For this review, take the finished solid that the model builds, in its own axes (mm). Give positions to 0.01 mm unless a question says otherwise; leave off trailing zeros. Order: outer loops, then holes, each group sorted by start corner. A loop starts at its lowest first (then second) coordinate and runs counter-clockwise, first axis right, second up. Notation, with made-up numbers: M -23.75,-20 L -2.75,-20 A18 ccw -2.75,14 Z; hole C -34,-39.75 d5. An arc over 180 degrees is marked long. Use CSV: the item, a comma, the result in double quotes. Start each with the question number.
(1) Clearance check with flat-ended pins moving along their axes: P1, Ø10, axis at x = 5, y = -5.5, coming from the -Z side; P2, Ø4, axis at x = -8.5, z = 75, coming from the -Y side; P3, Ø4.5, axis at x = -14, z = 120, coming from the -Y side; P4, Ø3, axis at x = -2.5, y = 4.5, coming from the -Z side. State where each tip first meets the part, or that it passes through.
(2) Consider section C-C (z = 33). Write out the cut boundary in (x, y).
(3) Consider section B-B (x = 2.25). Write out the cut boundary in (y, z).
(4) Consider section A-A (z = 84.5). Write out the cut boundary in (x, y).
(5) Wall thickness on L1, parallel to Z at x = -9.5, y = -2.5; L2, parallel to Z at x = -11.25, y = 0.75; L3, parallel to X at y = 0, z = 160.5: over which ranges is each line inside the solid? List them lowest first. Write a range as from..to.
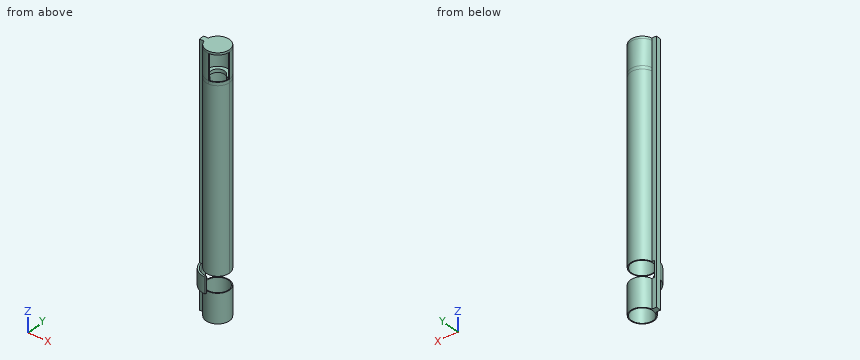
```python
from build123d import *
from build123d.topology import SkipClean

# Parameters (mm, degrees)
SCHIZZO1_R                  = 11
SCHIZZO1_R_2                = 10.15
TUBO_DEPTH                  = 210
INGRESSOCAVI_DEPTH          = 27
SCHIZZO4_R                  = 11
SCHIZZO4_R_2                = 6.5
FONDOCORSA_DEPTH            = 3
SCHIZZO5_R                  = 11
TAPPO_DEPTH                 = 2
BASEINFERIORE_DEPTH         = 239
SCHIZZO7_R                  = 13.5
TAGLIOANELLO_DEPTH          = 15
SUPPORTOANELLO_DEPTH        = 15
FACILITAZIONECAVI_DEPTH     = 3
RACCORDOFACILITAZIONECAVI_R = 8


with BuildPart() as part:
    # Schizzo1 → Tubo (new body)
    with BuildSketch(Plane.XY):
        Circle(SCHIZZO1_R)
        Circle(SCHIZZO1_R_2, mode=Mode.SUBTRACT)
    extrude(amount=TUBO_DEPTH)

    # Schizzo2 → IngressoCavi (add)
    with BuildSketch(Plane.XY.offset(210)):
        with BuildLine():
            Line((0, -10.15), (0, -11))
            ThreePointArc((0, -11), (-7.778174593, 7.778174593), (11, 0))
            Line((11, 0), (10.15, 0))
            ThreePointArc((10.15, 0), (-7.177133829, 7.177133829), (0, -10.15))
        make_face()
    extrude(amount=INGRESSOCAVI_DEPTH)

    # Schizzo4 → FondoCorsa (add)
    with SkipClean():  # the faces are left unmerged after this step: merging them gives an invalid solid
        with BuildSketch(Plane.XY.offset(210)):
            Circle(SCHIZZO4_R)
            Circle(SCHIZZO4_R_2, mode=Mode.SUBTRACT)
        extrude(amount=FONDOCORSA_DEPTH)

    # Schizzo5 → Tappo (add)
    with SkipClean():  # the faces are left unmerged after this step: merging them gives an invalid solid
        with BuildSketch(Plane.XY.offset(237)):
            Circle(SCHIZZO5_R)
        extrude(amount=TAPPO_DEPTH)
    add(part.part.scale(1), mode=Mode.REPLACE)  # the faces are merged on a copy

    # Schizzo6 → BaseInferiore (add)
    with SkipClean():  # the faces are left unmerged after this step: merging them gives an invalid solid
        with BuildSketch(Plane.XY):
            Polygon((-11, 2.5), (-15, 2.5), (-15, -2.5), (-11, -2.5), (-10.712142643, -2.5), (-10.712142643, 2.5), align=None)
        extrude(amount=BASEINFERIORE_DEPTH)

    # Schizzo7 → TaglioAnello (cut)
    with BuildSketch(Plane.XY.offset(27)):
        Circle(SCHIZZO7_R)
    extrude(amount=TAGLIOANELLO_DEPTH, mode=Mode.SUBTRACT)

    # Schizzo8 → SupportoAnello (add)
    with SkipClean():  # the faces are left unmerged after this step: merging them gives an invalid solid
        with BuildSketch(Plane.XY.offset(27)):
            with BuildLine():
                Line((-15, 0), (-13.5, 0))
                ThreePointArc((-13.5, 0), (-9.545941546, -9.545941546), (0, -13.5))
                Line((0, -13.5), (0, -15))
                ThreePointArc((0, -15), (-10.606601718, -10.606601718), (-15, 0))
            make_face()
        extrude(amount=SUPPORTOANELLO_DEPTH)

    # Schizzo9 → FacilitazioneCavi (cut)
    with SkipClean():  # the faces are left unmerged after this step: merging them gives an invalid solid
        with BuildSketch(Plane(origin=(0, 0, 210), x_dir=(-1, 0, 0), z_dir=(0, 0, -1))):
            with BuildLine():
                Line((-10.15, 0), (0, 0))
                Line((0, 0), (0, -10.15))
                ThreePointArc((0, -10.15), (-7.177133829, -7.177133829), (-10.15, 0))
            make_face()
        extrude(amount=-FACILITAZIONECAVI_DEPTH, mode=Mode.SUBTRACT)

    # RaccordoFacilitazioneCavi
    # the kernel refuses this fillet: 8 mm, written as the material it takes off along each edge
    with BuildSketch(Plane(origin=(0, -6.5, 222.125), x_dir=(0, -1, 0), z_dir=(0, 0, -1)), Plane(origin=(6.5, 0, 200.875), x_dir=(1, 0, 0), z_dir=(0, 0, 1))) as raccordofacilitazionecavi_piece_1:
        with BuildLine():
            CenterArc((5.779433498, 7.711388525), RACCORDOFACILITAZIONECAVI_R, 212.128500683, 42.43446725)
            Line((-0.995426363, 3.456829339), (-1.13092356, 3.371738155))
            ThreePointArc((-1.13092356, 3.371738155), (-0.407564337, 1.754373873), (-0.16, 0))
            Line((-0.16, 0), (0, -0.16))
            ThreePointArc((0, -0.16), (1.825, -0.16), (3.60741133, -0.15422777))
            Line((3.60741133, -0.15422777), (3.65, 0))
        make_face()
    extrude(amount=21.25, mode=Mode.SUBTRACT)


solid = part.part
```
Check result:
1,P1,"stops at z = 0"
1,P2,"stops at y = -8.87"
1,P3,"stops at y = -2.5"
1,P4,"stops at z = 210"
2,outline,"M -15,-2.5 L -14.79,-2.5 A15 ccw 0,-15 L 0,-13.5 A13.5 cw -13.27,2.5 L -15,2.5 Z"
3,outline,"M -10.77,0 L -9.9,0 L -9.9,27 L -10.77,27 Z; M -10.77,42 L -9.9,42 L -9.9,213 L -10.77,213 Z; M -10.77,237 L 9.9,237 L 9.9,213 L 6.1,213 L 6.1,210 L 9.9,210 L 9.9,42 L 10.77,42 L 10.77,239 L -10.77,239 Z; M 9.9,0 L 10.77,0 L 10.77,27 L 9.9,27 Z"
4,outline,"M -15,-2.5 L -10.71,-2.5 A11 ccw long -10.71,2.5 L -15,2.5 Z; hole C 0,0 d20.3"
5,L1,"z = 210..213, 237..239"
5,L2,"z = 0..27, 42..239"
5,L3,"x = -15..-10.15, 10.15..11"
